from build123d import *

# Parameters (mm, degrees)
SKETCH_1_R          = 28.5
SKETCH_1_R_2        = 21
EXTRUDE_1_DEPTH     = 2
SKETCH_2_R          = 1.2
CUT_EXTRUDE_1_DEPTH = 41.354677548
HOLE_WIZARD_M2_1_D  = 2.4


with BuildPart() as part:
    # 스케치1 → 보스-돌출1 (new body)
    with BuildSketch(Plane.XY):
        Circle(SKETCH_1_R)
        Circle(SKETCH_1_R_2, mode=Mode.SUBTRACT)
    extrude(amount=EXTRUDE_1_DEPTH)

    # 스케치2 → 컷-돌출1 (cut, through all)
    with BuildSketch(Plane.XY):
        with Locations((0, 25.455844123)):
            Circle(SKETCH_2_R)
        with Locations((25.455844123, 0)):
            Circle(SKETCH_2_R)
        with Locations((-25.455844123, 0)):
            Circle(SKETCH_2_R)
        with Locations((0, -25.455844123)):
            Circle(SKETCH_2_R)
    extrude(amount=CUT_EXTRUDE_1_DEPTH, mode=Mode.SUBTRACT)

    # M2 여유 구멍1 (through all)
    with Locations(Plane(origin=(-17, 17, 2), x_dir=(1, 0, 0), z_dir=(0, 0, 1))):
        with Locations((0, 0), (34, 0), (34, -34), (0, -34)):
            Hole(HOLE_WIZARD_M2_1_D / 2)


solid = part.part
Could you check a few things on this model? Use its own coordinates, in mm. Give positions to 0.01 mm unless a question says otherwise; leave off trailing zeros. Order: outer loops, then holes, each group sorted by start corner. A loop starts at its lowest first (then second) coordinate and runs counter-clockwise, first axis right, second up.
Item 1: If we section it at A-A, the plane y = -4.5: Write out the boundary of the cut face in (x, z).
Item 2: If we section it at C-C, the plane z = 1.6: Count the separate pieces of the cut face and the enclosed holes in it, plus the area to 3 significant figures.
Item 3: If we mould it in two halves opening along X, with no side actions, what happens to faces 1 (the face through (-24.31, 0.36, 0.99)), 2 (the face through (-15, 15, 2)), 3 (the face through (26.327, -10.916, 0.986))? For each: pulls with the +X half, pulls with the -X half, needs draft (parallel to the pull), parting line crosses it, or undercut.
Item 4: If we section it at B-B, the plane x = -8: Write out the boundary of the cut face in (y, z).
Item 5: I need wall thicknesses on line 1 (Y direction, x = 0, z = 0.6); line 2 (Y direction, x = -17, z = 0.8); line 3 (X direction, y = 0.5, z = 0.9). Which ranges of each line are inside material? Lowest first, please.
Item 6: I'm going to push flat-ended pins straight in: pin 1 (3 mm diameter, centred on x = 0, y = -25.46, fed in from +Z); pin 2 (1 mm diameter, centred on x = -22.5, z = 1, fed in from +Y). Where does each tip first touch, or does it pass through?
Item 7: If we section it at D-D, the plane x = 0: Write out the boundary of the cut face in (y, z).
Values:
1. outline: (-28.14, 0) - (-20.51, 0) - (-20.51, 2) - (-28.14, 2) - close; (20.51, 0) - (28.14, 0) - (28.14, 2) - (20.51, 2) - close
2. separate pieces: 1
2. enclosed holes: 9
2. area: 1,130 mm2
3. face 1: undercut
3. face 2: needs draft
3. face 3: parting line crosses it
4. outline: (-27.35, 0) - (-19.42, 0) - (-19.42, 2) - (-27.35, 2) - close; (19.42, 0) - (27.35, 0) - (27.35, 2) - (19.42, 2) - close
5. line 1: y = -28.5 to -26.66, -24.26 to -21, 21 to 24.26, 26.66 to 28.5
5. line 2: y = -22.87 to -18.2, -15.8 to -12.33, 12.33 to 15.8, 18.2 to 22.87
5. line 3: x = -28.5 to -26.55, -24.36 to -20.99, 20.99 to 24.36, 26.55 to 28.5
6. pin 1: stops at z = 2
6. pin 2: stops at y = 18.12
7. outline: (-28.5, 0) - (-26.66, 0) - (-26.66, 2) - (-28.5, 2) - close; (-24.26, 0) - (-21, 0) - (-21, 2) - (-24.26, 2) - close; (21, 0) - (24.26, 0) - (24.26, 2) - (21, 2) - close; (26.66, 0) - (28.5, 0) - (28.5, 2) - (26.66, 2) - close
